```python
from build123d import *

# Parameters (mm, degrees)
F0_R      = 21.1455
F2_R      = 25.0825
F4_DEPTH  = 34.544
F6_R      = 13.97
F4_FACE_R = 25.0825
F8_R      = 8.001
F9_DEPTH  = 4.318
F10_R     = 3.00355
F11_DEPTH = 15.24
F12_R     = 6.0325
F13_DEPTH = 4.064
F14_R     = 2.9845
F15_DEPTH = 2.794
F16_R     = 2.15265
F17_DEPTH = 4.953
F18_R     = 2.15265
F18_R_2   = 7.0485
F19_DEPTH = 4.064
F20_R     = 8.5725
F21_DEPTH = 10.414
F22_R     = 9.525
F23_DEPTH = 1.651
F24_R     = 7.9375
F25_DEPTH = 12.7
F26_R     = 9.525
F27_DEPTH = 1.651
F29_DEPTH = 6.35


# Not quite as in the source:
# - a feature names something its author has since deleted; it is built from what else it names


with BuildPart() as f3:
    # F0 (on Top) → F3 section 0
    with BuildSketch(Plane.XY):
        Circle(F0_R)
    # F2 (on offset) → F3 section 1
    with BuildSketch(Plane.XY.offset(16.129)):
        Circle(F2_R)
    loft()

    # F4 (add): a face of the model
    f4_faces = [f3.faces().sort_by_distance(p)[0] for p in [
        (0, 0, 16.129),
    ]]
    extrude(f4_faces, amount=F4_DEPTH)

    # F6 (on offset) → F7 section 0
    with BuildSketch(Plane.XY.offset(57.023)):
        Circle(F6_R)
    # F4_face (on face) → F7 section 1
    with BuildSketch(Plane.XY.offset(50.673)):
        Circle(F4_FACE_R)
    loft()

    # F8 (on face) → F9 (join)
    with BuildSketch(Plane.XY.offset(57.023)):
        Circle(F8_R)
    extrude(amount=F9_DEPTH)

    # F10 (on face) → F11 (join)
    with BuildSketch(Plane.XY.offset(61.341)):
        Circle(F10_R)
    extrude(amount=F11_DEPTH)

    # F12 (on face) → F13 (join)
    with BuildSketch(Plane(origin=(0, 0, 0), x_dir=(1, 0, 0), z_dir=(0, 0, -1))):
        Circle(F12_R)
    extrude(amount=F13_DEPTH)

    # F14 (on face) → F15 (join)
    with BuildSketch(Plane(origin=(0, 0, -4.064), x_dir=(1, 0, 0), z_dir=(0, 0, -1))):
        Circle(F14_R)
    extrude(amount=F15_DEPTH)

    # F16 (on face) → F17 (cut)
    with BuildSketch(Plane(origin=(0, 0, 0), x_dir=(1, 0, 0), z_dir=(0, 0, -1))):
        with Locations((0, 13.26515)):
            Circle(F16_R)
        with Locations((13.26515, 0)):
            Circle(F16_R)
        with Locations((0, -13.26515)):
            Circle(F16_R)
        with Locations((-13.26515, 0)):
            Circle(F16_R)
    extrude(amount=-F17_DEPTH, mode=Mode.SUBTRACT)

    # F18 (on face) → F19 (join)
    with BuildSketch(Plane(origin=(0, 0, 0), x_dir=(1, 0, 0), z_dir=(0, 0, -1))):
        with BuildLine():
            ThreePointArc((11.557, 5.207), (7.0668719395, 7.0668719395), (5.207, 11.557))
            Line((5.207, 11.557), (5.207, 29.01315))
            ThreePointArc((5.207, 29.01315), (0, 34.22015), (-5.207, 29.01315))
            Line((-5.207, 29.01315), (-5.207, 11.557))
            ThreePointArc((-5.207, 11.557), (-7.0668719395, 7.0668719395), (-11.557, 5.207))
            Line((-11.557, 5.207), (-29.01315, 5.207))
            ThreePointArc((-29.01315, 5.207), (-34.22015, 0), (-29.01315, -5.207))
            Line((-29.01315, -5.207), (-11.557, -5.207))
            ThreePointArc((-11.557, -5.207), (-7.0668719395, -7.0668719395), (-5.207, -11.557))
            Line((-5.207, -11.557), (-5.207, -29.01315))
            ThreePointArc((-5.207, -29.01315), (0, -34.22015), (5.207, -29.01315))
            Line((5.207, -29.01315), (5.207, -11.557))
            ThreePointArc((5.207, -11.557), (7.0668719395, -7.0668719395), (11.557, -5.207))
            Line((11.557, -5.207), (29.01315, -5.207))
            ThreePointArc((29.01315, -5.207), (34.22015, 0), (29.01315, 5.207))
            Line((29.01315, 5.207), (11.557, 5.207))
        make_face()
        with Locations((0, -29.01315)):
            Circle(F18_R, mode=Mode.SUBTRACT)
        with Locations((0, -13.26515)):
            Circle(F18_R, mode=Mode.SUBTRACT)
        with Locations((-29.01315, 0)):
            Circle(F18_R, mode=Mode.SUBTRACT)
        with Locations((-13.26515, 0)):
            Circle(F18_R, mode=Mode.SUBTRACT)
        Circle(F18_R_2, mode=Mode.SUBTRACT)
        with Locations((13.26515, 0)):
            Circle(F18_R, mode=Mode.SUBTRACT)
        with Locations((0, 13.26515)):
            Circle(F18_R, mode=Mode.SUBTRACT)
        with Locations((29.01315, 0)):
            Circle(F18_R, mode=Mode.SUBTRACT)
        with Locations((0, 29.01315)):
            Circle(F18_R, mode=Mode.SUBTRACT)
    extrude(amount=F19_DEPTH)

    # F20 (on face) → F21 (join)
    with BuildSketch(Plane.XY.offset(61.341)):
        Circle(F20_R)
    extrude(amount=F21_DEPTH)

    # F22 (on face) → F23 (join)
    with BuildSketch(Plane.XY.offset(71.755)):
        Circle(F22_R)
    extrude(amount=F23_DEPTH)

    # F24 (on face) → F25 (join)
    with BuildSketch(Plane.XY.offset(73.406)):
        Circle(F24_R)
    extrude(amount=F25_DEPTH)

    # F26 (on face) → F27 (join)
    with BuildSketch(Plane.XY.offset(86.106)):
        Circle(F26_R)
    extrude(amount=F27_DEPTH)

    # F28 (on face) → F29 (join)
    with BuildSketch(Plane.XY.offset(87.757)):
        Polygon((6.6499638915, 8.760449774), (-4.2617901071, 10.1392625512), (-10.9117539986, 1.3788127773), (-6.6499638915, -8.760449774), (4.2617901071, -10.1392625512), (10.9117539986, -1.3788127773), align=None)
    extrude(amount=F29_DEPTH)


solid = f3.part
```
Verification items for the finished model (mm, model axes). A direction names the side the tool comes from. Coordinates: 2 decimals unless noted, no trailing zeros. Order: outer loops, then holes, each group sorted by start corner. A loop starts at its lowest first (then second) coordinate and runs counter-clockwise, first axis right, second up. Notation, with made-up numbers: (2, 17) -> (27, 17) arc R4 cw to (27, 21) -> close; hole circle Ø9 at (-36.75, -14). An arc over 180 degrees is marked (long way). Put each result on its own line as item: value. Start each with the question number.
1) Release check for a two-part mould opening along Y. For faces 5 (the flat face through (-2, 8, 73.406)), 6 (the cylindrical face through (-5.593, 4.289, -2.004)), 7 (the cylindrical face through (-7.559, -5.796, 86.92)) record: pulls with the +Y half, pulls with the -Y half, needs draft (parallel to the pull), parting line crosses it, or undercut.
2) Cross-section at D-D (z = 7.5). Enter the section's corners in (x, y).
3) Cross-section at B-B (x = 0). State how many separate pieces and enclosed holes the cut face has, plus the area to 3 significant figures.
4) Tool access check on faces 1 (the flat face through (6, -6, 57.023)), 2 (the flat face through (7.4, -0.2, -4.064)), 3 (the cylindrical face through (7.117, -7.018, -2.004)), 4 (the flat face through (1.27, 9.44, 90.89)). Record the directions out of +Z, -Z, +X, -X, +Y, -Y that give a thin tool (end or side, any length) a straight path to the whole face; none if there is none.
5) Material ranges on L1, parallel to Y at x = 0, z = 0.5; L2, parallel to X at y = 0, z = 2; L3, parallel to Y at x = 0, z = 2.5, recorded low to high.
6) Cross-section at A-A (z = 81). Enter the section's corners in (x, y) (1 decimal).
7) Go/stop test with flat-tipped pins: pin 1 (8 mm diameter, centred on x = 21, y = -25, fed in from +Z); pin 2 (2 mm diameter, centred on y = -22, z = -3, fed in from -X); pin 3 (1 mm diameter, centred on y = -0.5, z = 12.5, fed in from +X); pin 4 (8.5 mm diameter, centred on x = 26.5, y = 0, fed in from +Z). Record where each tip stops, or that it passes through.
Geometry check:
1. face 5: needs draft
1. face 6: undercut
1. face 7: parting line crosses it
2. outline: circle Ø45.95 at (0, 0)
3. separate pieces: 3
3. enclosed holes: 0
3. area: 3,530 mm^2
4. face 1: none
4. face 2: -Z
4. face 3: -Z, +X, -Y
4. face 4: +Z, +X, +Y
5. L1: y = -21.27 to -15.42, -11.11 to 11.11, 15.42 to 21.27
5. L2: x = -21.63 to -15.42, -11.11 to 11.11, 15.42 to 21.63
5. L3: y = -21.76 to -15.42, -11.11 to 11.11, 15.42 to 21.76
6. outline: circle Ø15.9 at (0, 0)
7. pin 1: passes through
7. pin 2: stops at x = -5.21
7. pin 3: stops at x = 24.31
7. pin 4: stops at z = 52.29
